from build123d import *

# Parameters (mm, degrees)
Y_KSEKLIK_EKSTR_ZYON1_DEPTH = 14
KES_EKSTR_ZYON1_DEPTH       = 33.044227249
KES_EKSTR_ZYON3_DEPTH       = 33.044227249
KES_EKSTR_ZYON4_START       = -4.4
KES_EKSTR_ZYON4_DEPTH       = 4.4
KES_EKSTR_ZYON6_REACH       = 48.442
IZIM6_R                     = 3.6
IZIM5_R                     = 1.6
KES_EKSTR_ZYON5_DEPTH       = 37.282674929
KES_EKSTR_ZYON7_DEPTH       = 2.2
KES_EKSTR_ZYON8_REACH       = 46.576
IZIM7_R                     = 0.6
KES_EKSTR_ZYON10_REACH      = 48.442
IZIM9_R                     = 3.5
IZIM9_3_R                   = 4.75
IZIM9_3_R_2                 = 3.5
KES_EKSTR_ZYON11_DEPTH      = 4
RADYUS1_R                   = 2
IZIM5_3_R                   = 4
KES_EKSTR_ZYON12_DEPTH      = 3
PAH1_SIZE                   = 1.5


# Read off the part's stored shape, not the designer's step: Kes-Ekstrüzyon4
with BuildPart() as part:
    # Çizim1 → Yükseklik-Ekstrüzyon1 (new, symmetric)
    with BuildSketch(Plane(origin=(0, 0, 0), x_dir=(1, 0, 0), z_dir=(0, 1, 0))):
        Polygon((-19.85, -7), (-19.85, 20.9), (19.85, 20.9), (19.85, -7), (15.45, -7), (15.45, 16.5), (-15.45, 16.5), (-15.45, -7), align=None)
    extrude(amount=Y_KSEKLIK_EKSTR_ZYON1_DEPTH, both=True)

    # Çizim2 → Kes-Ekstrüzyon1 (cut, through all)
    with BuildSketch(Plane(origin=(0, 0, 0), x_dir=(0, 0, -1), z_dir=(1, 0, 0))):
        with BuildLine():
            Line((20.9, -12), (-1.571984828, -6.821206909))
            ThreePointArc((-1.571984828, -6.821206909), (-5.477403299, -4.358675613), (-7, 0))
            Line((-7, 0), (-7, -14))
            Line((-7, -14), (20.9, -14))
            Line((20.9, -14), (20.9, -12))
        make_face()
        with BuildLine():
            Line((-7, 14), (-7, 0))
            ThreePointArc((-7, 0), (-5.477403299, 4.358675613), (-1.571984828, 6.821206909))
            Line((-1.571984828, 6.821206909), (20.9, 12))
            Line((20.9, 12), (20.9, 14))
            Line((20.9, 14), (-7, 14))
        make_face()
    extrude(amount=-KES_EKSTR_ZYON1_DEPTH, mode=Mode.SUBTRACT)

    # Çizim3 → Kes-Ekstrüzyon3 (cut, through all)
    with BuildSketch(Plane(origin=(0, 0, 0), x_dir=(0, 0, -1), z_dir=(1, 0, 0))):
        with BuildLine():
            ThreePointArc((-7, 3e-09), (-5.477403298, 4.358675614), (-1.571984828, 6.821206909))
            Line((-1.571984828, 6.821206909), (20.9, 12))
            Line((20.9, 12), (20.9, 14))
            Line((20.9, 14), (-7, 14))
            Line((-7, 14), (-7, 3e-09))
        make_face()
        with BuildLine():
            ThreePointArc((-1.571984828, -6.821206909), (-5.4774033, -4.358675612), (-7, 3e-09))
            Line((-7, 3e-09), (-7, -14))
            Line((-7, -14), (20.9, -14))
            Line((20.9, -14), (20.9, -12))
            Line((20.9, -12), (-1.571984828, -6.821206909))
        make_face()
    extrude(amount=KES_EKSTR_ZYON3_DEPTH, mode=Mode.SUBTRACT)

    # Kes-Ekstrüzyon4 outline → Kes-Ekstrüzyon4 (cut)
    with BuildSketch(Plane.XY.offset(-16.5).offset(KES_EKSTR_ZYON4_START)):
        with BuildLine():
            Line((-19.85, 10.985995684), (-15.45, 10.985995684))
            ThreePointArc((-15.45, 10.985995684), (-10.259984059, 11.487506015), (-5.262018305, 12.973479231))
            ThreePointArc((-5.262018305, 12.973479231), (-2.680605384, 13.740973574), (5.9e-08, 14))
            Line((5.9e-08, 14), (-19.85, 14))
            Line((-19.85, 14), (-19.85, 10.985995684))
        make_face()
        with BuildLine():
            ThreePointArc((-5.262018305, -12.973479231), (-10.259984059, -11.487506015), (-15.45, -10.985995684))
            Line((-15.45, -10.985995684), (-19.85, -10.985995684))
            Line((-19.85, -10.985995684), (-19.85, -14))
            Line((-19.85, -14), (0, -14))
            ThreePointArc((0, -14), (-2.680605414, -13.740973569), (-5.262018305, -12.973479231))
        make_face()
        with BuildLine():
            Line((19.85, 14), (5.9e-08, 14))
            ThreePointArc((5.9e-08, 14), (2.680605443, 13.740973563), (5.262018305, 12.973479231))
            ThreePointArc((5.262018305, 12.973479231), (10.259984059, 11.487506015), (15.45, 10.985995684))
            Line((15.45, 10.985995684), (19.85, 10.985995684))
            Line((19.85, 10.985995684), (19.85, 14))
        make_face()
        with BuildLine():
            ThreePointArc((5.262018305, -12.973479231), (2.680605414, -13.740973569), (0, -14))
            Line((0, -14), (19.85, -14))
            Line((19.85, -14), (19.85, -10.985995684))
            Line((19.85, -10.985995684), (15.45, -10.985995684))
            ThreePointArc((15.45, -10.985995684), (10.259984059, -11.487506015), (5.262018305, -12.973479231))
        make_face()
    extrude(amount=KES_EKSTR_ZYON4_DEPTH, mode=Mode.SUBTRACT)

    # Çizim6 → Kes-Ekstrüzyon6 (cut, up to next)
    with BuildSketch(Plane(origin=(19.85, 0, 0), x_dir=(0, 0, -1), z_dir=(1, 0, 0)), mode=Mode.PRIVATE) as kes_ekstr_zyon6_sk1:
        Circle(IZIM6_R)
    kes_ekstr_zyon6_tool1 = extrude(kes_ekstr_zyon6_sk1.sketch, amount=-KES_EKSTR_ZYON6_REACH, mode=Mode.PRIVATE) & part.part
    add(kes_ekstr_zyon6_tool1.solids().sort_by_distance((19.85, 0, 0))[0], mode=Mode.SUBTRACT)

    # Çizim5 → Kes-Ekstrüzyon5 (cut, through all)
    with BuildSketch(Plane(origin=(0, 0, -20.9), x_dir=(-1, 0, 0), z_dir=(0, 0, -1))):
        with Locations((-5.656854249, -5.656854249)):
            Circle(IZIM5_R)
        with Locations((-6.717514421, 6.717514421)):
            Circle(IZIM5_R)
        with Locations((5.656854249, 5.656854249)):
            Circle(IZIM5_R)
        with Locations((6.717514421, -6.717514421)):
            Circle(IZIM5_R)
    extrude(amount=-KES_EKSTR_ZYON5_DEPTH, mode=Mode.SUBTRACT)

    # Çizim6<3> → Kes-Ekstrüzyon7 (cut)
    with BuildSketch(Plane(origin=(19.85, 0, 0), x_dir=(0, 0, -1), z_dir=(1, 0, 0))):
        with BuildLine():
            ThreePointArc((0.297744361, 3.587666135), (3.6, 0), (0.297744361, -3.587666135))
            Line((0.297744361, -3.587666135), (13.506766917, -2.491434816))
            ThreePointArc((13.506766917, -2.491434816), (15.8, 0), (13.506766917, 2.491434816))
            Line((13.506766917, 2.491434816), (0.297744361, 3.587666135))
        make_face()
    extrude(amount=-KES_EKSTR_ZYON7_DEPTH, mode=Mode.SUBTRACT)

    # Çizim7 → Kes-Ekstrüzyon8 (cut, up to next)
    with BuildSketch(Plane(origin=(17.65, 0, 0), x_dir=(0, 0, -1), z_dir=(1, 0, 0)), mode=Mode.PRIVATE) as kes_ekstr_zyon8_sk1:
        with Locations((13.3, 0)):
            Circle(IZIM7_R)
    kes_ekstr_zyon8_tool1 = extrude(kes_ekstr_zyon8_sk1.sketch, amount=-KES_EKSTR_ZYON8_REACH, mode=Mode.PRIVATE) & part.part
    add(kes_ekstr_zyon8_tool1.solids().sort_by_distance((17.65, 0, -13.3))[0], mode=Mode.SUBTRACT)

    # Çizim9 → Kes-Ekstrüzyon10 (cut, up to next)
    with BuildSketch(Plane.ZY.offset(19.85), mode=Mode.PRIVATE) as kes_ekstr_zyon10_sk1:
        Circle(IZIM9_R)
    kes_ekstr_zyon10_tool1 = extrude(kes_ekstr_zyon10_sk1.sketch, amount=-KES_EKSTR_ZYON10_REACH, mode=Mode.PRIVATE) & part.part
    add(kes_ekstr_zyon10_tool1.solids().sort_by_distance((-19.85, 0, 0))[0], mode=Mode.SUBTRACT)

    # Çizim9<3> → Kes-Ekstrüzyon11 (cut)
    with BuildSketch(Plane.ZY.offset(19.85)):
        Circle(IZIM9_3_R)
        Circle(IZIM9_3_R_2, mode=Mode.SUBTRACT)
    extrude(amount=-KES_EKSTR_ZYON11_DEPTH, mode=Mode.SUBTRACT)

    # Radyus1
    # the kernel refuses this fillet: 2 mm, written as the material it adds along each edge
    with BuildSketch(Plane(origin=(-15.45, -15.985995684, -16.5), x_dir=(0, 0, 1), z_dir=(0, 1, 0))) as radyus1_piece_1_section:
        with BuildLine():
            CenterArc((RADYUS1_R, RADYUS1_R), RADYUS1_R, 180, 90)
            Line((0, RADYUS1_R), (0, 0))
            Line((0, 0), (RADYUS1_R, 0))
        make_face()
    radyus1_piece_1 = extrude(amount=31.971991369, mode=Mode.PRIVATE)
    radyus1_piece_1 = split(radyus1_piece_1, bisect_by=Plane(origin=(-14.994883818, 10.333733048, -13.66968108), z_dir=(0, -0.9744581299008602, -0.22456926118709647)), keep=Keep.TOP, mode=Mode.PRIVATE)
    radyus1_piece_1 = split(radyus1_piece_1, bisect_by=Plane(origin=(-14.994883818, -10.333733048, -13.66968108), z_dir=(0, 0.9744581299008602, -0.22456926118709647)), keep=Keep.TOP, mode=Mode.PRIVATE)
    add(radyus1_piece_1)
    with BuildSketch(Plane(origin=(15.45, 15.985995684, -16.5), x_dir=(-1, 0, 0), z_dir=(0, -1, 0))) as radyus1_piece_2_section:
        with BuildLine():
            CenterArc((RADYUS1_R, -RADYUS1_R), RADYUS1_R, 90, 90)
            Line((0, -RADYUS1_R), (0, 0))
            Line((0, 0), (RADYUS1_R, 0))
        make_face()
    radyus1_piece_2 = extrude(amount=31.971991369, mode=Mode.PRIVATE)
    radyus1_piece_2 = split(radyus1_piece_2, bisect_by=Plane(origin=(14.994883818, -10.333733048, -13.66968108), z_dir=(0, 0.9744581299008602, -0.22456926118709647)), keep=Keep.TOP, mode=Mode.PRIVATE)
    radyus1_piece_2 = split(radyus1_piece_2, bisect_by=Plane(origin=(14.994883818, 10.333733048, -13.66968108), z_dir=(0, -0.9744581299008602, -0.22456926118709647)), keep=Keep.TOP, mode=Mode.PRIVATE)
    add(radyus1_piece_2)
    # the kernel refuses this fillet: 2 mm, written as the material it takes off along each edge
    with BuildSketch(Plane(origin=(-19.85, 15.985995684, -20.9), x_dir=(0, 0, 1), z_dir=(0, -1, 0)), Plane(origin=(19.85, 15.985995684, -20.9), x_dir=(-1, 0, 0), z_dir=(0, -1, 0))) as radyus1_2_piece_1:
        with BuildLine():
            CenterArc((RADYUS1_R, -RADYUS1_R), RADYUS1_R, 90, 90)
            Line((0, -RADYUS1_R), (0, 0))
            Line((0, 0), (RADYUS1_R, 0))
        make_face()
    extrude(amount=31.971991368, mode=Mode.SUBTRACT)

    # Çizim5<3> → Kes-Ekstrüzyon12 (cut)
    with BuildSketch(Plane(origin=(0, 0, -20.9), x_dir=(-1, 0, 0), z_dir=(0, 0, -1))):
        Circle(IZIM5_3_R)
    extrude(amount=-KES_EKSTR_ZYON12_DEPTH, mode=Mode.SUBTRACT)

    # Pah1
    pah1_edges = [part.edges().sort_by_distance(p)[0] for p in [
        (4, 0, -17.9),
    ]]
    chamfer(pah1_edges, length=PAH1_SIZE)


solid = part.part
CAD build for the part. Positions are in the model's coordinates, mm. A direction names the side the tool comes from. Coordinates: 2 decimals unless noted, no trailing zeros. Write each loop counter-clockwise with the first axis right and the second up, starting at its lowest first coordinate (ties: lowest second). Pieces come first, ordered by that corner, then holes. Notation, with made-up numbers: M -17.75,75 L 13.25,75 A28 cw 13.25,95 Z; hole C -0.5,24.25 d5. An arc over 180 degrees is marked long. Return JSON: item names as keys, results as strings.
Item 1: Slice it at D-D, the plane x = -10.5. Write the cut outline in (y, z).
Findings below:
{"outline": "M -11.44,-20.9 L 11.44,-20.9 L 11.44,-18.48 L 10.99,-16.5 L -10.99,-16.5 L -11.44,-18.48 Z"}
Item 2: Slice it at A-A, the plane z = 2.25. Write the cut outline in (x, y), and give its area (3 significant figures).
Findings below:
{"outline": "M -19.85,-6.63 L -15.45,-6.63 L -15.45,-2.68 L -15.85,-2.68 L -15.85,-4.18 L -19.85,-4.18 Z; M -19.85,4.18 L -15.85,4.18 L -15.85,2.68 L -15.45,2.68 L -15.45,6.63 L -19.85,6.63 Z; M 15.45,-6.63 L 19.85,-6.63 L 19.85,-2.81 L 15.45,-2.81 Z; M 15.45,2.81 L 19.85,2.81 L 19.85,6.63 L 15.45,6.63 Z", "area": "56.3 mm2"}
Item 3: Drop flat-ended pins along their axis: pin 1 Ø6.5 at (y, z) = (0, 0) entering from -X; pin 2 Ø4 at (x, y) = (0, 0) entering from -Z; pin 3 Ø3.5 at (y, z) = (0, -8) entering from +X; pin 4 Ø2 at (x, z) = (-16.5, -18.5) entering from -Y. Give the stop position or say it passes through.
Findings below:
{"pin 1": "passes through", "pin 2": "stops at z = -17.9", "pin 3": "stops at x = 17.65", "pin 4": "stops at y = -10.99"}
Item 4: Which spindle directions (+Z, -Z, +X, -X, +Y, -Y) get a long thin tool onto all of the face, cutting with end or side? Do faces 1 (the flat face through (18, 10.986, -19)), 2 (the flat face through (15.45, 0, -6)), 3 (the flat face through (-18, 10.986, -19)), 4 (the flat face through (18.765, -3.047, -6.81)). Say none if no direction does.
Findings below:
{"face 1": "+Z, -Z, +X, +Y", "face 2": "+Z, +Y, -Y", "face 3": "+Z, -Z, -X, +Y", "face 4": "+X"}
Item 5: Probe line 1 (X direction, y = 9, z = -10.5); line 2 (Z direction, x = -2.5, y = -9.25); line 3 (Y direction, x = -15.5, z = -17.25). List the from-to ranges inside material, lowest first. Write a range as from..to.
Findings below:
{"line 1": "x = -19.85..-15.45, 15.45..19.85", "line 2": "z = -20.9..-16.5", "line 3": "y = -10.99..10.99"}
Item 6: Slice it at B-B, the plane x = 0. Write the cut outline in (y, z), and give its area (3 significant figures).
Findings below:
{"outline": "M -12,-20.9 L -4,-20.9 L -4,-19.4 L -2.5,-17.9 L 2.5,-17.9 L 4,-19.4 L 4,-20.9 L 12,-20.9 L 10.99,-16.5 L -10.99,-16.5 Z", "area": "79.4 mm2"}
Item 7: Slice it at C-C, the plane z = -6. Write the cut outline in (x, y).
Findings below:
{"outline": "M -19.85,-8.57 L -15.45,-8.57 L -15.45,8.57 L -19.85,8.57 Z; M 15.45,-8.57 L 19.85,-8.57 L 19.85,-3.11 L 17.65,-3.11 L 17.65,3.11 L 19.85,3.11 L 19.85,8.57 L 15.45,8.57 Z"}
Item 8: Two-plate mould, pull along Y, no slides. Class faces 5 (the flat face through (0, 0, -17.9)), 6 (the flat face through (18, -10.986, -19)), 7 (the flat face through (-4.2, 0.2, -20.9)), 8 (the cylindrical face through (18.8, -0.1, -15.8)): +Y half, -Y half, draft (parallel to the pull), parting line (faces both ways), or undercut.
Findings below:
{"face 5": "undercut", "face 6": "-Y half", "face 7": "draft", "face 8": "undercut"}
